Check sheet for the modelled part. Datum: model origin and axes. Units: mm. Round coordinates to 2 decimals unless told otherwise and drop trailing zeros. Write each loop counter-clockwise with the first axis right and the second up, starting at its lowest first coordinate (ties: lowest second). Pieces come first, ordered by that corner, then holes. Notation, with made-up numbers: (31.25, -40) -> (67.25, -40) arc R21 ccw to (67.25, -19) -> close; hole circle Ø1 at (2.25, -19.75). An arc over 180 degrees is marked (long way). One line per item, written item: value.
Autodesk Inventor part; units mm, degrees
ref_plane "YZ Plane" through (0, 0, 0) normal (1, 0, 0) x (0, 1, 0)
ref_plane "XZ Plane" through (0, 0, 0) normal (0, 1, 0) x (-1, 0, 0)
ref_plane "XY Plane" through (0, 0, 0) normal (0, 0, 1) x (1, 0, 0)
sketch "Szkic1" plane through (0, 0, 0) normal (0, 0, 1) x (1, 0, 0)
  line L0 (-10.3866, 5.557) -> (25.6134, 5.557)
  line L1 (25.6134, 5.557) -> (25.6134, -36.443)
  line L2 (25.6134, -36.443) -> (-10.3866, -36.443)
  line L3 (-10.3866, -36.443) -> (-10.3866, 5.557)
  point P0 (0, 0)
  point P1 (20.6134, -0.193)
  point P2 (20.6134, -30.693)
  point P3 (-5.3866, -0.193)
  point P4 (-5.3866, -30.693)
  dimension "d0" = 36
  dimension "d1" = 42
  dimension "d2" = 5
  dimension "d3" = 5
  dimension "d4" = 5
  dimension "d5" = 5
  dimension "d6" = 5.75
  dimension "d7" = 5.75
  dimension "d8" = 5.75
  dimension "d9" = 5.75
extrude "Wyciągnięcie proste1" add sketch "Szkic1" along normal blind 7.55
hole "Otwór1" at (20.6134, -0.193, 0) at (20.6134, -30.693, 0) at (-5.3866, -0.193, 0) at (-5.3866, -30.693, 0) direction (0, 0, 1) diameter 5 end through all
sketch "Szkic2" plane through (-10.3866, -36.443, 0) normal (0, -1, 0) x (1, 0, 0)
  line L0 (36, 0) -> (0, 0)
  line L1 (36, 0) -> (36, 7.55)
  line L2 (0, 7.55) -> (36, 7.55)
  line L3 (0, 0) -> (0, 7.55)
  line L4 (36, 7.55) -> (0, 7.55)
  circle A0 centre (18, 7.55) radius 5.05
  point P0 (10.3866, 0)
  dimension "d19" = 36
  dimension "d20" = 18
  dimension "d21" = 10.1
extrude "Wyciągnięcie proste2" cut sketch "Szkic2" against normal through all contours A0 L2 | L2 A0
fillet "Zaokrąglenie1" radius 1 4 edges at (-10.3866, -36.443, 3.775) (-10.3866, 5.557, 3.775) (25.6134, -36.443, 3.775) (25.6134, 5.557, 3.775)
properties part number "3DP_ABS_X_Axis_Linear_Shaft_Clamp_Base"
Item 1: Depth check by flat-ended pin: P1, Ø4, axis at x = 10, y = -8, coming from the +Z side. Enter the tip coordinate at first touch or a pass-through.
Answer:
P1: stops at z = 5.05
Item 2: Sectioned sample at B-B on x = 22. Enter the section's corners in (y, z), and give its area (3 significant figures).
Answer:
outline: (-36.44, 0) -> (-32.77, 0) -> (-32.77, 7.55) -> (-36.44, 7.55) -> close; (-28.61, 0) -> (-2.27, 0) -> (-2.27, 7.55) -> (-28.61, 7.55) -> close; (1.89, 0) -> (5.56, 0) -> (5.56, 7.55) -> (1.89, 7.55) -> close
area: 254 mm^2
Item 3: Sectioned sample at D-D on y = -6.5. Enter the section's corners in (x, z).
Answer:
outline: (-10.39, 0) -> (25.61, 0) -> (25.61, 7.55) -> (12.66, 7.55) arc R5.05 cw to (2.56, 7.55) -> (-10.39, 7.55) -> close
Item 4: Sectioned sample at C-C on z = 6. Enter the section's corners in (x, y).
Answer:
outline: (-10.39, -35.44) arc R1 ccw to (-9.39, -36.44) -> (2.81, -36.44) -> (2.81, 5.56) -> (-9.39, 5.56) arc R1 ccw to (-10.39, 4.56) -> close; (12.42, -36.44) -> (24.61, -36.44) arc R1 ccw to (25.61, -35.44) -> (25.61, 4.56) arc R1 ccw to (24.61, 5.56) -> (12.42, 5.56) -> close; hole circle Ø5 at (-5.39, -30.69); hole circle Ø5 at (-5.39, -0.19); hole circle Ø5 at (20.61, -30.69); hole circle Ø5 at (20.61, -0.19)
Item 5: Sectioned sample at A-A on z = 3. Enter the section's corners in (x, y), and give its area (3 significant figures).
Answer:
outline: (-10.39, -35.44) arc R1 ccw to (-9.39, -36.44) -> (5.42, -36.44) -> (5.42, 5.56) -> (-9.39, 5.56) arc R1 ccw to (-10.39, 4.56) -> close; (9.8, -36.44) -> (24.61, -36.44) arc R1 ccw to (25.61, -35.44) -> (25.61, 4.56) arc R1 ccw to (24.61, 5.56) -> (9.8, 5.56) -> close; hole circle Ø5 at (-5.39, -30.69); hole circle Ø5 at (-5.39, -0.19); hole circle Ø5 at (20.61, -30.69); hole circle Ø5 at (20.61, -0.19)
area: 1,250 mm^2
Item 6: Thickness scan on line 1 (X direction, y = 0, z = 2); line 2 (X direction, y = -2, z = 1.25); line 3 (X direction, y = -29, z = 5.25). Record the ranges inside material, lowest first.
Answer:
line 1: x = -10.39 to -7.88, -2.89 to 18.12, 23.11 to 25.61
line 2: x = -10.39 to -7.11, -3.66 to 18.89, 22.34 to 25.61
line 3: x = -10.39 to -7.23, -3.55 to 3.12, 12.11 to 18.77, 22.45 to 25.61
Item 7: Mould release check, pull along X, two halves, no side actions. Record for faces 1 (the cylindrical face through (23.054, -0.735, 3.828)), 2 (the flat face through (8, -36.443, 2)), 3 (the cylindrical face through (-10.101, -36.142, 3.828)): pulls with the +X half, pulls with the -X half, needs draft (parallel to the pull), parting line crosses it, or undercut.
Answer:
face 1: undercut
face 2: needs draft
face 3: pulls with the -X half
